The figure shows three views and two pictorial views of one solid part (mm, origin at its lowest corner). Answer the questions. A direction names the side the tool comes from. Round coordinates to 2 decimals unless told otherwise and drop trailing zeros. Order: outer loops, then holes, each group sorted by start corner. A loop starts at its lowest first (then second) coordinate and runs counter-clockwise, first axis right, second up. Notation, with made-up numbers: (-2.75, 39) - (28.25, 39) arc R22 cw to (28.25, 55) - close; hole circle Ø9 at (40, 58). An arc over 180 degrees is marked (long way). Answer in a Markdown table with one row per item.
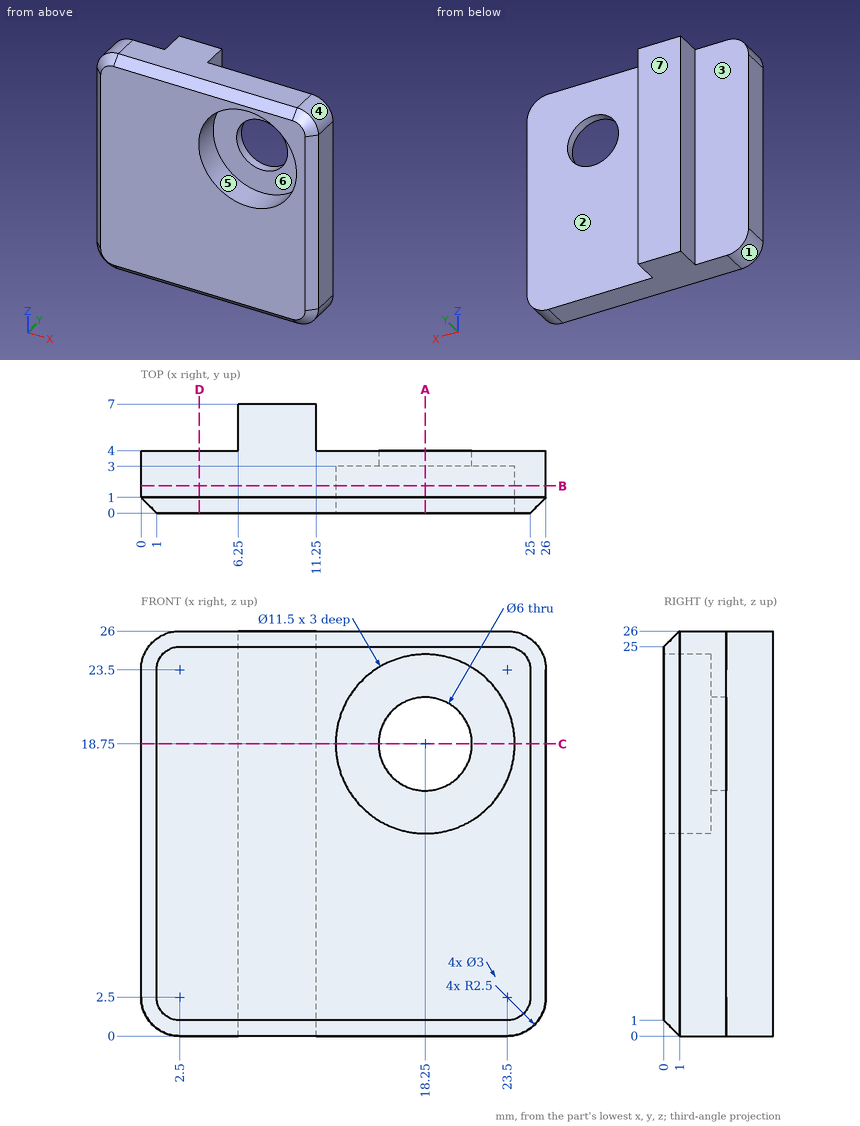
1) Find section C-C, the plane z = 18.75. Give the vertices of the cut face in (x, y).
Filled in:
| item | result |
|---|---|
| outline | (0, 1) - (1, 0) - (12.5, 0) - (12.5, 3) - (15.25, 3) - (15.25, 4) - (11.25, 4) - (11.25, 7) - (6.25, 7) - (6.25, 4) - (0, 4) - close; (21.25, 3) - (24, 3) - (24, 0) - (25, 0) - (26, 1) - (26, 4) - (21.25, 4) - close |
2) Which of the six approach directions +Z, -Z, +X, -X, +Y, -Y give full straight-line access (tool end or side, diameter ignored) to the marked faces 1, 2 and 3?
Filled in:
| item | result |
|---|---|
| face 1 | -Z, -X, +Y, -Y |
| face 2 | +Z, -Z, +X, +Y |
| face 3 | +Z, -Z, -X, +Y |
3) Find section D-D, the plane x = 3.75. Give the vertices of the cut face in (y, z).
Filled in:
| item | result |
|---|---|
| outline | (0, 1) - (1, 0) - (4, 0) - (4, 26) - (1, 26) - (0, 25) - close |
4) Find section A-A, the plane x = 18.25. Give the vertices of the cut face in (y, z).
Filled in:
| item | result |
|---|---|
| outline | (0, 1) - (1, 0) - (4, 0) - (4, 15.75) - (3, 15.75) - (3, 13) - (0, 13) - close; (0, 24.5) - (3, 24.5) - (3, 21.75) - (4, 21.75) - (4, 26) - (1, 26) - (0, 25) - close |
5) Find section B-B, the plane y = 1.75. Give the vertices of the cut face in (x, z).
Filled in:
| item | result |
|---|---|
| outline | (0, 2.5) arc R2.5 ccw to (2.5, 0) - (23.5, 0) arc R2.5 ccw to (26, 2.5) - (26, 23.5) arc R2.5 ccw to (23.5, 26) - (2.5, 26) arc R2.5 ccw to (0, 23.5) - close; hole circle Ø11.5 at (18.25, 18.75) |
6) Find the intervals of material crossed by probe 1 along Z at (x, y) = (18.25, 3.3); probe 2 along Y at (x, z) = (23, 10.25); probe 3 along X at (y, z) = (4.25, 17.25), in increasing order. Write a range as from..to.
Filled in:
| item | result |
|---|---|
| probe 1 | z = 0..15.75, 21.75..26 |
| probe 2 | y = 0..4 |
| probe 3 | x = 6.25..11.25 |
7) Each of these flat-tipped pins is pushed along its axis until it touches: pin 1 (9 mm diameter, centred on x = 18.25, z = 18.75, fed in from +Y); pin 2 (0.9 mm diameter, centred on y = 5, z = 11.5, fed in from +X); pin 3 (3.5 mm diameter, centred on y = 6, z = 14, fed in from -X). Where does it stop, or does it pass through?
Filled in:
| item | result |
|---|---|
| pin 1 | stops at y = 4 |
| pin 2 | stops at x = 11.25 |
| pin 3 | stops at x = 6.25 |
8) The mould has two halves that part along X. Classify the marked faces 4, 5, 6 and 7: released by +X, released by -X, zero draft, split by the parting line, or undercut.
Filled in:
| item | result |
|---|---|
| face 4 | released by +X |
| face 5 | undercut |
| face 6 | undercut |
| face 7 | zero draft |
